For this review, use the dimensioned drawing (mm, ordinates from the lowest corner) and the shaded views. A direction names the side the tool comes from. Give positions to 0.01 mm unless a question says otherwise; leave off trailing zeros. Loops run counter-clockwise (first coordinate to the right, second up) from the corner with the lowest first, then second, coordinate; pieces in that order, holes last. Notation, with made-up numbers: M -36,34.5 L -20,34.5 A21 cw -20,57.5 Z; hole C 75,29 d2. An arc over 180 degrees is marked long. Use one line per item in the form item = value. Start each with the question number.
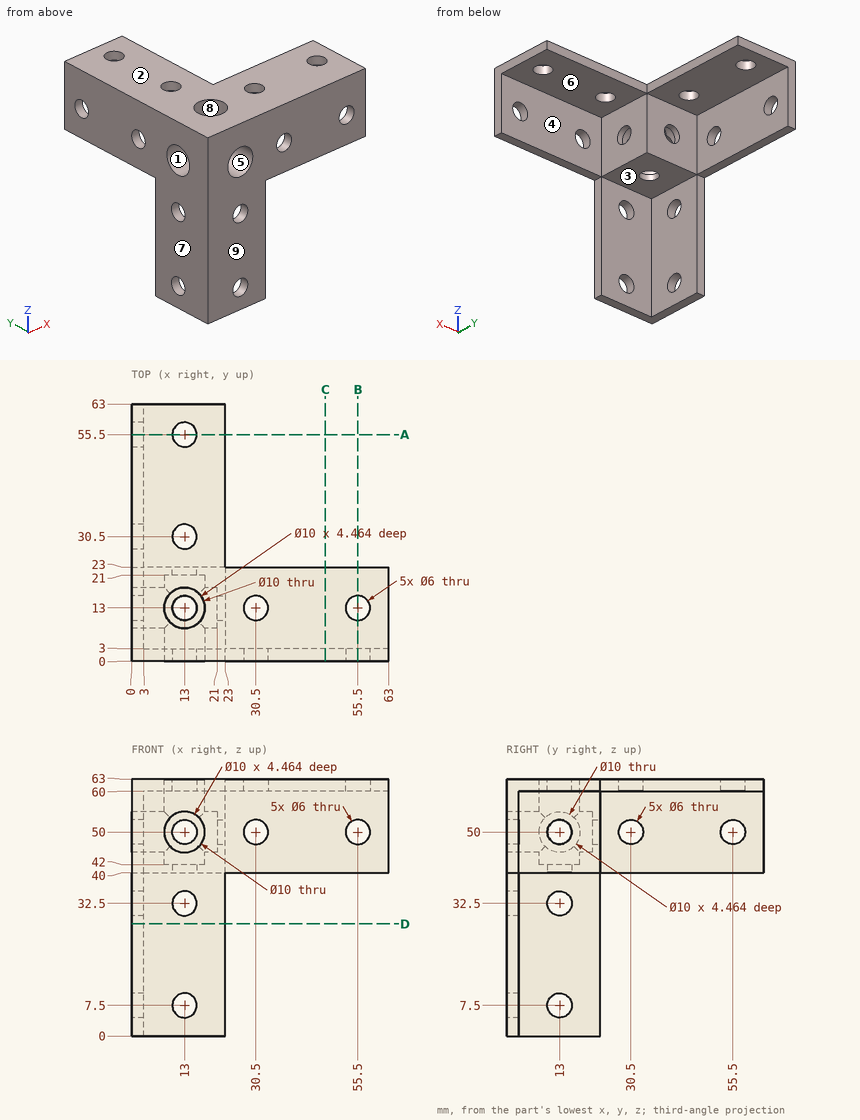
Q1. Take a section at D-D on z = 27.5. Give the boundary of the cut face in (x, y), plus the area to 3 significant figures.
Q2. The part is to be moulded in two halves that separate along Z. For the marked faces 1, 2, 3 and 4, say which applies: pulls with the +Z half, pulls with the -Z half, needs draft (parallel to the pull), parting line crosses it, or undercut.
Q3. Take a section at A-A on y = 55.5. Give the boundary of the cut face in (x, z).
Q4. Wall thickness on probe 1 along Z at (x, y) = (22, 13); probe 2 along Y at (x, z) = (6, 50); probe 3 along X at (y, z) = (46, 56): over which ranges is each line inside the solid? List them lowest first.
Q5. For the marked faces 5, 6, 7, 8 and 9, list the 3-axis set-ups (+Z, -Z, +X, -X, +Y, -Y) from which the entire face can be reached by the end or side of a thin tool; tool diameter is ignored.
Q6. Clearance check with flat-ended pins moving along their axes: pin 1 Ø10 at (x, y) = (9.5, 16) entering from -Z; pin 2 Ø0.9 at (x, z) = (33.5, 61.5) entering from +Y; pin 3 Ø9.5 at (x, z) = (13, 32.5) entering from +Y; pin 4 Ø5 at (x, y) = (13, 13) entering from -Z. State where each tip first meets the part, or that it passes through.
Q7. Take a section at C-C on x = 47.5. Give the boundary of the cut face in (y, z).
Response values:
q1.outline = M 0,0 L 23,0 L 23,3 L 3,3 L 3,23 L 0,23 Z
q1.area = 129 mm^2
q2.face_1 = undercut
q2.face_2 = pulls with the +Z half
q2.face_3 = pulls with the -Z half
q2.face_4 = needs draft
q3.outline = M 0,40 L 3,40 L 3,47 L 0,47 Z; M 0,53 L 3,53 L 3,60 L 10,60 L 10,63 L 0,63 Z; M 16,60 L 23,60 L 23,63 L 16,63 Z
q4.probe_1 = 40 to 47, 53 to 63
q4.probe_2 = 0 to 8, 18 to 23
q4.probe_3 = 0 to 3
q5.face_5 = -Y
q5.face_6 = -Z, +X, +Y
q5.face_7 = +Z, -Z, -X, +Y, -Y
q5.face_8 = +Z
q5.face_9 = +Z, -Z, +X, -X, -Y
q6.pin_1 = 40
q6.pin_2 = 23
q6.pin_3 = 3
q6.pin_4 = through
q7.outline = M 0,40 L 3,40 L 3,60 L 23,60 L 23,63 L 0,63 Z
